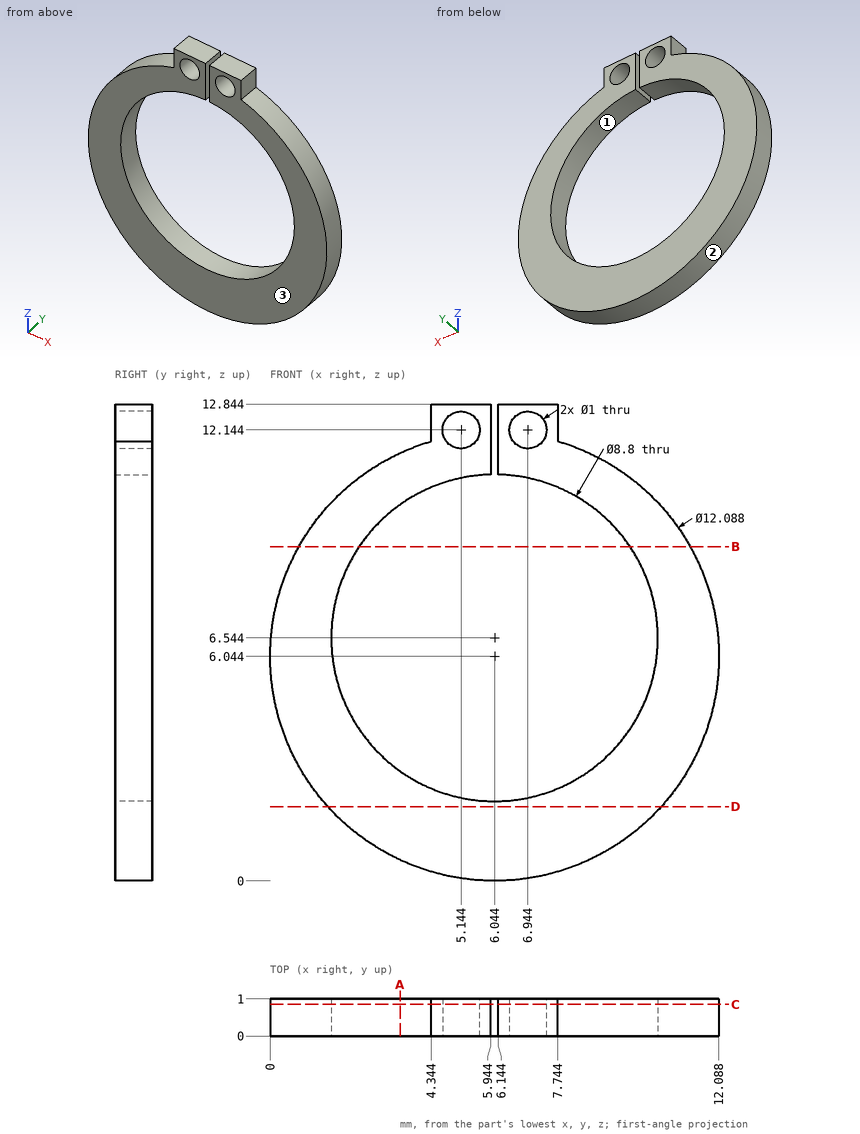
Check sheet for the drawn part. Datum: minimum x, y, z corner. Units: mm. Coordinates: 2 decimals unless noted, no trailing zeros. Write each loop counter-clockwise with the first axis right and the second up, starting at its lowest first coordinate (ties: lowest second). Pieces come first, ordered by that corner, then holes. Notation, with made-up numbers: (49, 74.25) - (55, 74.25) arc R31 cw to (55, 112.25) - close; hole circle Ø7 at (17, 6). An arc over 180 degrees is marked (long way). Answer as a JSON object with one key per item and string values.
(1) Cross-section at B-B on z = 9. Record the cut outline in (x, y), plus the area to 3 significant figures.
Report:
{"outline": "(0.77, 0) - (2.39, 0) - (2.39, 1) - (0.77, 1) - close; (9.69, 0) - (11.32, 0) - (11.32, 1) - (9.69, 1) - close", "area": "3.24 mm^2"}
(2) Mould release check, pull along X, two halves, no side actions. Record for the marked faces 1, 2 and 3: pulls with the +X half, pulls with the -X half, needs draft (parallel to the pull), parting line crosses it, or undercut.
Report:
{"face 1": "undercut", "face 2": "parting line crosses it", "face 3": "needs draft"}
(3) Cross-section at C-C on y = 0.85. Record the cut outline in (x, z), plus the area to 3 significant figures.
Report:
{"outline": "(4.34, 11.84) arc R6.04 ccw (long way) to (7.74, 11.84) - (7.74, 12.84) - (6.14, 12.84) - (6.14, 10.94) arc R4.4 cw (long way) to (5.94, 10.94) - (5.94, 12.84) - (4.34, 12.84) - close; hole circle Ø1 at (5.14, 12.14); hole circle Ø1 at (6.94, 12.14)", "area": "54.8 mm^2"}
(4) Cross-section at D-D on z = 2. Record the cut outline in (x, y).
Report:
{"outline": "(1.55, 0) - (10.54, 0) - (10.54, 1) - (1.55, 1) - close"}
(5) Gauge pin test, flat end, axial feed: pin 1 Ø0.5 at (y, z) = (0.5, 12.5) entering from -X. Record the tip position at first contact, or that the pin passes through.
Report:
{"pin 1": "x = 4.34"}
(6) Thickness scan on line 1 along X through (y, z) = (0.5, 5.5); line 2 along X through (y, z) = (0.25, 6); line 3 along Z through (x, y) = (7, 0.95). Record the ranges inside material, lowest first.
Report:
{"line 1": "0.02 to 1.77, 10.32 to 12.06", "line 2": "0 to 1.68, 10.41 to 12.09", "line 3": "0.08 to 2.25, 10.84 to 11.65, 12.64 to 12.84"}
(7) Cross-section at A-A on x = 3.5. Record the cut outline in (y, z), plus the area to 4 significant figures.
Report:
{"outline": "(0, 0.56) - (1, 0.56) - (1, 2.95) - (0, 2.95) - close; (0, 10.13) - (1, 10.13) - (1, 11.53) - (0, 11.53) - close", "area": "3.785 mm^2"}
